The model under review builds one solid part; all positions refer to its coordinate system, in mm. A direction names the side the tool comes from. Give positions to 0.01 mm unless a question says otherwise; leave off trailing zeros. Write each loop counter-clockwise with the first axis right and the second up, starting at its lowest first coordinate (ties: lowest second). Pieces come first, ordered by that corner, then holes. Notation, with made-up numbers: M 44,-39.75 L 75,-39.75 A16 cw 75,-21.75 Z; hole C 84,-7 d8. An arc over 180 degrees is marked long. Write each question's results on one line, items separated by ' | '. Start each with the question number.
from build123d import *

# Parameters (mm, degrees)
BOSS_EXTRUDE1_DEPTH  = 75
SKETCH1_3_W          = 52.7
SKETCH1_3_H          = 18.9
BOSS_EXTRUDE2_DEPTH  = 3
CUT_EXTRUDE1_DEPTH   = 16.75
MIRROR3_COPY_1_DEPTH = 16.75
SKETCH5_W            = 15.25
SKETCH5_H            = 1.1
CUT_EXTRUDE2_DEPTH   = 2
FILLET1_R            = 3


with BuildPart() as part:
    # Sketch1 → Boss-Extrude1 (new body)
    with BuildSketch(Plane(origin=(0, 0, 0), x_dir=(1, 0, 0), z_dir=(0, 1, 0))):
        with BuildLine():
            Line((47.109992867, 3), (52.7, 3))
            Line((52.7, 3), (52.7, 11.15))
            Line((52.7, 11.15), (50.85, 11.15))
            ThreePointArc((50.85, 11.15), (49.870361389, 6.666414567), (47.109992867, 3))
        make_face()
        with BuildLine():
            Line((26.35, 11.15), (26.35, 3))
            Line((26.35, 3), (33.090007133, 3))
            ThreePointArc((33.090007133, 3), (30.329638611, 6.666414567), (29.35, 11.15))
            Line((29.35, 11.15), (26.35, 11.15))
        make_face()
        with BuildLine():
            Line((19.609992867, 3), (26.35, 3))
            Line((26.35, 3), (26.35, 11.15))
            Line((26.35, 11.15), (23.35, 11.15))
            ThreePointArc((23.35, 11.15), (22.370361389, 6.666414567), (19.609992867, 3))
        make_face()
        with BuildLine():
            Line((0, 3), (5.590007133, 3))
            ThreePointArc((5.590007133, 3), (2.829638611, 6.666414567), (1.85, 11.15))
            Line((1.85, 11.15), (0, 11.15))
            Line((0, 11.15), (0, 3))
        make_face()
    extrude(amount=BOSS_EXTRUDE1_DEPTH)

    # Sketch1<3> → Boss-Extrude2 (add)
    with BuildSketch(Plane(origin=(0, 0, 0), x_dir=(1, 0, 0), z_dir=(0, 1, 0))):
        with Locations((26.35, 12.45)):
            Rectangle(SKETCH1_3_W, SKETCH1_3_H)
    boss_extrude2 = extrude(amount=-BOSS_EXTRUDE2_DEPTH)

    # Sketch4 → Cut-Extrude1 (cut)
    with BuildSketch(Plane(origin=(0, 0, -21.9), x_dir=(-1, 0, 0), z_dir=(0, 0, -1))):
        Polygon((-18.725, -1.5), (-6.475, -1.5), (-6.475, -0.4), (-8.6, -0.4), (-8.6, 0), (-16.6, 0), (-16.6, -0.4), (-18.725, -0.4), align=None)
    cut_extrude1 = extrude(amount=-CUT_EXTRUDE1_DEPTH, mode=Mode.SUBTRACT)

    # Mirror2: Cut-Extrude1 across plane
    add(cut_extrude1.mirror(Plane(origin=(26.35, 0, 0), x_dir=(0, 0, 1), z_dir=(1, 0, 0))), mode=Mode.SUBTRACT)

    # Mirror3: Boss-Extrude2, Cut-Extrude1 across plane
    add(boss_extrude2.mirror(Plane.ZX.offset(37.5)))
    add(cut_extrude1.mirror(Plane.ZX.offset(37.5)), mode=Mode.SUBTRACT)

    # Mirror3 copy 1 sketch → Mirror3 copy 1 (cut)
    with BuildSketch(Plane(origin=(52.7, 75, -21.9), x_dir=(1, 0, 0), z_dir=(0, 0, -1))):
        Polygon((-18.725, -1.5), (-6.475, -1.5), (-6.475, -0.4), (-8.6, -0.4), (-8.6, 0), (-16.6, 0), (-16.6, -0.4), (-18.725, -0.4), align=None)
    extrude(amount=-MIRROR3_COPY_1_DEPTH, mode=Mode.SUBTRACT)

    # Sketch5 → Cut-Extrude2 (cut)
    with BuildSketch(Plane(origin=(0, 0, -21.9), x_dir=(-1, 0, 0), z_dir=(0, 0, -1))):
        with Locations((-26.35, 75.95)):
            Rectangle(SKETCH5_W, SKETCH5_H)
    extrude(amount=-CUT_EXTRUDE2_DEPTH, mode=Mode.SUBTRACT)

    # Fillet1
    fillet1_edges = [part.edges().sort_by_distance(p)[0] for p in [
        (0, 78, -12.45),
        (52.7, 78, -12.45),
        (52.7, -3, -12.45),
        (0, -3, -12.45),
    ]]
    fillet(fillet1_edges, radius=FILLET1_R - 0.0001)  # a hair under: the kernel refuses the full size


solid = part.part
(1) Add section A-A (x = 37.5). State the section outline as (y, z) points.
(2) Wall thickness on L1, parallel to X at y = 66, z = -10.5; L2, parallel to Y at x = 38, z = -8; L3, parallel to Y at x = 47.5, z = -5: over which ranges is each line inside the solid? List them lowest first.
(3) Add section B-B (y = 11.5). State the section outline as (x, z) points, then the cut area to 3 significant figures.
(4) Clearance check with flat-ended pins moving along their axes: P1, Ø0.8, axis at x = 12, y = 75.5, coming from the -Z side; P2, Ø4, axis at x = 27.5, y = 26, coming from the -Z side; P3, Ø0.6, axis at y = -1, z = -15, coming from the +X side; P4, Ø3, axis at x = 7.5, y = 8.5, coming from the +Z side. State where each tip first meets the part, or that it passes through.
(5) Machinability: for faces 1 (the flat face through (26, 0, -13)), 2 (the flat face through (52, 37, -11.15)), 3 (the flat face through (26, -3, -13)), which of the approach directions +Z, -Z, +X, -X, +Y, -Y give a long, thin tool a straight path to every point of the face, cutting with its end or side? Answer none if there is none.
(6) Add section C-C (z = -10.25). Give the number of separate pieces and of enclosed holes in the cut face, then the cut area to 3 significant figures.
(7) Draft analysis for pull direction X (two halves, no side actions). For faces 4 (the flat face through (25.6, 75.4, -20.4)), 5 (the flat face through (52.7, 37, -8)), 6 (the cylindrical face through (0.86, 77.1, -12.58)), 7 (the flat face through (1, 37, -11.15)), state which applies: pulls with the +X half, pulls with the -X half, needs draft (parallel to the pull), parting line crosses it, or undercut.
Calculated:
1) outline: M -3,-21.9 L -1.5,-21.9 L -1.5,-5.15 L 0,-5.15 L 0,-3 L -3,-3 Z; M 75,-5.15 L 76.5,-5.15 L 76.5,-21.9 L 78,-21.9 L 78,-3 L 75,-3 Z
2) L1: x = 0 to 1.87, 23.33 to 29.37, 50.83 to 52.7 | L2: y = -3 to -1.5, 76.5 to 78 | L3: y = -3 to 0, 75 to 78
3) outline: M 0,-11.15 L 1.85,-11.15 A10.75 cw 5.59,-3 L 0,-3 Z; M 19.61,-3 A10.75 cw 23.35,-11.15 L 29.35,-11.15 A10.75 cw 33.09,-3 Z; M 47.11,-3 A10.75 cw 50.85,-11.15 L 52.7,-11.15 L 52.7,-3 Z | area: 116 mm²
4) P1: stops at z = -5.15 | P2: stops at z = -11.15 | P3: stops at x = 52.62 | P4: passes through
5) face 1: -Z | face 2: -Z, +X, -X | face 3: +Z, -Z, +X, -X, -Y
6) separate pieces: 1 | enclosed holes: 2 | area: 981 mm²
7) face 4: undercut | face 5: pulls with the +X half | face 6: pulls with the -X half | face 7: needs draft
